from build123d import *

# Parameters (mm, degrees)
SKETCH1_W           = 43.20032
SKETCH1_H           = 28.39974
BOSS_EXTRUDE1_DEPTH = 13.4747
SKETCH2_W           = 33.20034
SKETCH2_H           = 20.39874
CUT_EXTRUDE1_DEPTH  = 10.2997
SKETCH3_W           = 5.19938
SKETCH3_H           = 12.10056
CUT_EXTRUDE2_DEPTH  = 53.715241631
BOSS_EXTRUDE2_DEPTH = 6.35
SKETCH5_W           = 6.35
SKETCH5_H           = 28.39974
BOSS_EXTRUDE3_DEPTH = 21.59
SKETCH6_R           = 9.25
CUT_EXTRUDE3_DEPTH  = 25.4
SKETCH7_R           = 0.9
CUT_EXTRUDE4_DEPTH  = 25.4
FILLET1_R           = 2.54
FILLET2_R           = 1.27
SKETCH8_R           = 1.651
CUT_EXTRUDE5_DEPTH  = 25.4


with BuildPart() as part:
    # Sketch1 → Boss-Extrude1 (new body)
    with BuildSketch(Plane(origin=(0, 0, 0), x_dir=(1, 0, 0), z_dir=(0, 1, 0))):
        with Locations((21.60016, 14.19987)):
            Rectangle(SKETCH1_W, SKETCH1_H)
    extrude(amount=BOSS_EXTRUDE1_DEPTH)

    # Sketch2 → Cut-Extrude1 (cut)
    with BuildSketch(Plane(origin=(0, 13.4747, 0), x_dir=(1, 0, 0), z_dir=(0, 1, 0))):
        with Locations((26.60015, 14.19987)):
            Rectangle(SKETCH2_W, SKETCH2_H)
    extrude(amount=-CUT_EXTRUDE1_DEPTH, mode=Mode.SUBTRACT)

    # Sketch3 → Cut-Extrude2 (cut, through all)
    with BuildSketch(Plane(origin=(0, 3.175, 0), x_dir=(1, 0, 0), z_dir=(0, 1, 0))):
        with Locations((17.60093, 14.19987)):
            Rectangle(SKETCH3_W, SKETCH3_H)
    extrude(amount=-CUT_EXTRUDE2_DEPTH, mode=Mode.SUBTRACT)

    # Sketch4 → Boss-Extrude2 (add)
    with BuildSketch(Plane(origin=(43.20032, 0, 0), x_dir=(0, 0, -1), z_dir=(1, 0, 0))):
        Polygon((24.39924, 3.175), (4.0005, 3.175), (4.0005, 13.4747), (0, 13.4747), (0, 0), (28.39974, 0), (28.39974, 13.4747), (24.39924, 13.4747), align=None)
    extrude(amount=BOSS_EXTRUDE2_DEPTH)

    # Sketch5 → Boss-Extrude3 (add)
    with BuildSketch(Plane(origin=(0, 3.175, 0), x_dir=(1, 0, 0), z_dir=(0, 1, 0))):
        with Locations((46.37532, 14.19987)):
            Rectangle(SKETCH5_W, SKETCH5_H)
    extrude(amount=BOSS_EXTRUDE3_DEPTH)

    # Sketch6 → Cut-Extrude3 (cut)
    with BuildSketch(Plane(origin=(49.55032, 0, 0), x_dir=(0, 0, -1), z_dir=(1, 0, 0))):
        with Locations((14.19987, 13.177)):
            Circle(SKETCH6_R)
    extrude(amount=-CUT_EXTRUDE3_DEPTH, mode=Mode.SUBTRACT)

    # Sketch7 → Cut-Extrude4 (cut)
    with BuildSketch(Plane(origin=(49.55032, 0, 0), x_dir=(0, 0, -1), z_dir=(1, 0, 0))):
        with Locations((6.49987, 21.039)):
            Circle(SKETCH7_R)
        with Locations((21.89987, 21.039)):
            Circle(SKETCH7_R)
        with Locations((21.89987, 5.639)):
            Circle(SKETCH7_R)
        with Locations((6.49987, 5.639)):
            Circle(SKETCH7_R)
    extrude(amount=-CUT_EXTRUDE4_DEPTH, mode=Mode.SUBTRACT)

    # Fillet1
    fillet1_edges = [part.edges().sort_by_distance(p)[0] for p in [
        (46.37532, 24.765, -28.39974),
        (46.37532, 24.765, 0),
    ]]
    fillet(fillet1_edges, radius=FILLET1_R)

    # Fillet2
    fillet2_edges = [part.edges().sort_by_distance(p)[0] for p in [
        (21.60016, 13.4747, -28.39974),
        (0, 13.4747, -14.19987),
        (21.60016, 13.4747, 0),
    ]]
    fillet(fillet2_edges, radius=FILLET2_R)

    # Sketch8 → Cut-Extrude5 (cut)
    with BuildSketch(Plane(origin=(0, 13.4747, 0), x_dir=(1, 0, 0), z_dir=(0, 1, 0))):
        with Locations(Location((5.63499, 21.6675, 0), (0, 0, 270))):
            Circle(SKETCH8_R)
        with Locations(Location((5.63499, 6.6675, 0), (0, 0, 270))):
            Circle(SKETCH8_R)
    extrude(amount=-CUT_EXTRUDE5_DEPTH, mode=Mode.SUBTRACT)


solid = part.part
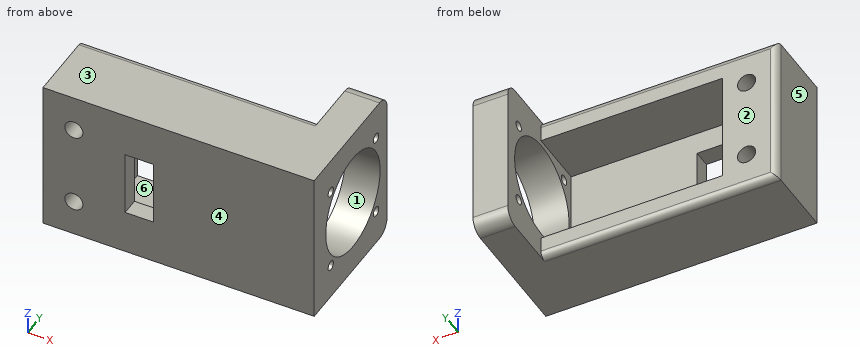
Input: part model. Units: mm. Frame: model coordinates. Face numbers are marked on the shaded views. A direction names the side the tool comes from. Give positions to 0.01 mm unless a question says otherwise; leave off trailing zeros. Loops run counter-clockwise (first coordinate to the right, second up) from the corner with the lowest first, then second, coordinate; pieces in that order, holes last. Notation, with made-up numbers: M 68.5,31.25 L 98.5,31.25 A20 ccw 98.5,46.25 Z; hole C 15.5,5 d10. An arc over 180 degrees is marked long. Use one line per item in the form item = value.
1. Pull-direction query (Y, two-part tool) for the marked faces 1, 2, 3 and 4; classes: released by +Y, released by -Y, zero draft, split by the parting line, or undercut.
Numbers:
face_1 = undercut
face_2 = released by +Y
face_3 = zero draft
face_4 = released by -Y
2. Line query: L1, parallel to Z at x = 31, y = 3.25; L2, parallel to X at y = 1.75, z = -9.75; L3, parallel to Z at x = 17.5, y = 2.5. Output: solid intervals per line, ascending.
Numbers:
L1 = -28.4 to -24.4, -4 to 0
L2 = 0 to 15, 20.2 to 49.55
L3 = -28.4 to -20.25, -8.15 to 0
3. Section query B-B, the plane z = -14.5. Return the cut outline in (x, y) (3 decimals).
Numbers:
outline = M 0,0 L 15.001,0 L 15.001,3.175 L 10,3.175 L 10,13.475 L 1.27,13.475 A1.27 ccw 0,12.205 Z; M 20.201,0 L 49.55,0 L 49.55,3.932 L 43.2,3.932 L 43.2,3.175 L 20.201,3.175 Z; M 43.2,22.422 L 49.55,22.422 L 49.55,24.765 L 43.2,24.765 Z
4. Section query A-A, the plane z = -21.5. Return the cut outline in (x, y) (1 decimal), and give its area (3 significant figures).
Numbers:
outline = M 0,0 L 4,0 L 4,13.5 L 1.3,13.5 A1.3 ccw 0,12.2 Z; M 7.3,0 L 49.6,0 L 49.6,4.8 L 43.2,4.8 L 43.2,3.2 L 10,3.2 L 10,13.5 L 7.3,13.5 Z; M 43.2,6.4 L 49.6,6.4 L 49.6,7.5 L 43.2,7.5 Z; M 43.2,18.9 L 49.6,18.9 L 49.6,20.2 L 43.2,20.2 Z; M 43.2,21.8 L 49.6,21.8 L 49.6,24.8 L 43.2,24.8 Z
area = 260 mm²
5. Section query D-D, the plane y = 10. Return the cut outline in (x, z) (1 decimal), and give its area (3 significant figures).
Numbers:
outline = M 0,-28.4 L 49.6,-28.4 L 49.6,-22.9 L 43.2,-22.9 L 43.2,-24.4 L 10,-24.4 L 10,-4 L 43.2,-4 L 43.2,-5.5 L 49.6,-5.5 L 49.6,0 L 0,0 Z; hole C 5.6,-21.7 d3.3; hole C 5.6,-6.7 d3.3
area = 603 mm²
6. Section query C-C, the plane x = 12. Return the cut outline in (y, z) (1 decimal).
Numbers:
outline = M 0,-28.4 L 12.2,-28.4 A1.3 ccw 13.5,-27.1 L 13.5,-24.4 L 3.2,-24.4 L 3.2,-4 L 13.5,-4 L 13.5,-1.3 A1.3 ccw 12.2,0 L 0,0 Z
7. Reachability of the marked faces 5 and 6 from +Z, -Z, +X, -X, +Y, -Y: full face, straight path, thin tool, end or side. Return the list, or none.
Numbers:
face_5 = +Z, -Z, -X, +Y, -Y
face_6 = +Y
8. First-contact query: pin 1 (13 mm diameter, centred on x = 16, z = -16, fed in from +Y); pin 2 (1.4 mm diameter, centred on y = 5.64, z = -6.5, fed in from +X); pin 3 (1.1 mm diameter, centred on y = 21.04, z = -21.9, fed in from -X); pin 4 (6 mm diameter, centred on x = 31, z = -19, fed in from +Y) (3 decimals). Flat tips, straight axial feed; report the tip coordinate or a pass-through.
Numbers:
pin_1 = 13.47
pin_2 = 10
pin_3 = through
pin_4 = 3.175
